Drawing for the job (mm, zero at the part's lowest x, y, z). A direction names the side the tool comes from. Give positions to 0.01 mm unless a question says otherwise; leave off trailing zeros. Order: outer loops, then holes, each group sorted by start corner. A loop starts at its lowest first (then second) coordinate and runs counter-clockwise, first axis right, second up. Notation, with made-up numbers: M 20.25,9.25 L 79.25,9.25 A29 cw 79.25,41.25 Z; hole C -23.5,14 d6. An arc over 180 degrees is marked long. One line per item, written item: value.
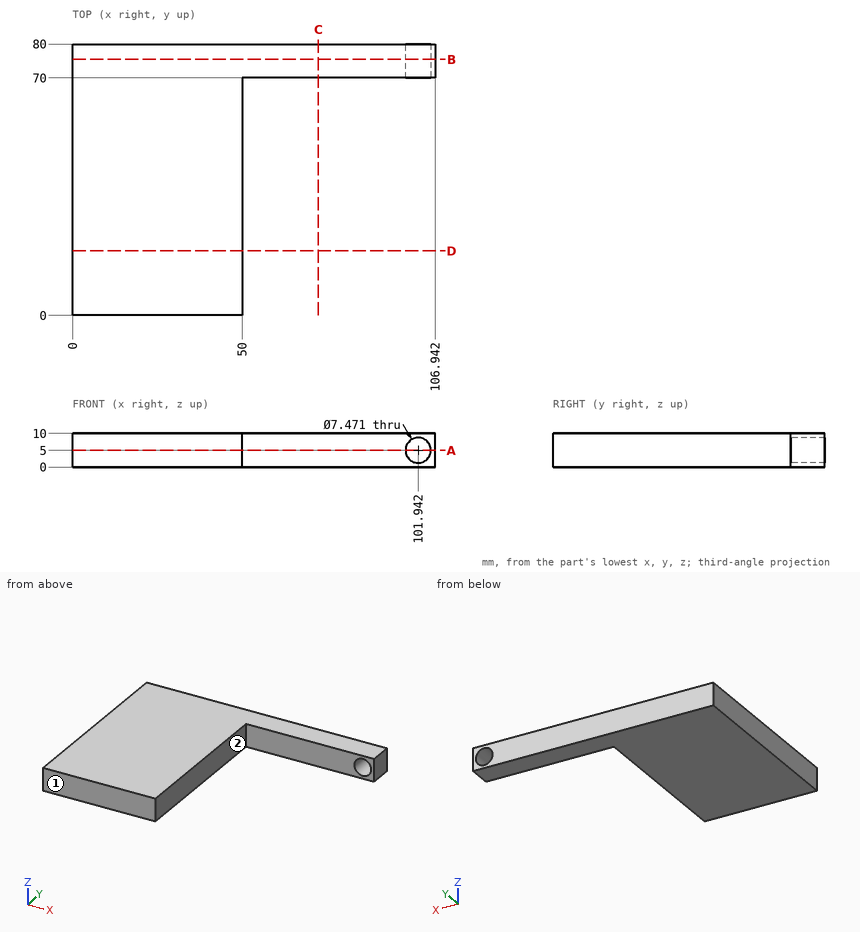
1) Saw through at B-B, the plane y = 75.5. Write the cut outline in (x, z) (1 decimal).
Check values:
outline: M 0,0 L 106.9,0 L 106.9,10 L 0,10 Z; hole C 101.9,5 d7.5
2) Saw through at D-D, the plane y = 19. Write the cut outline in (x, z), then the cut area to 3 significant figures.
Check values:
outline: M 0,0 L 50,0 L 50,10 L 0,10 Z
area: 500 mm^2
3) Saw through at C-C, the plane x = 72.5. Write the cut outline in (y, z), then the cut area to 3 significant figures.
Check values:
outline: M 70,0 L 80,0 L 80,10 L 70,10 Z
area: 100 mm^2
4) Pin check, flat tips, straight feed: pin 1 (1.5 mm diameter, centred on x = 38.5, y = 53.5, fed in from -Z); pin 2 (5 mm diameter, centred on x = 90.5, z = 5.5, fed in from -Y); pin 3 (4 mm diameter, centred on y = 13, z = 4.5, fed in from +X). Stop position of each tip, or through.
Check values:
pin 1: z = 0
pin 2: y = 70
pin 3: x = 50
5) Saw through at A-A, the plane z = 5. Write the cut outline in (x, y).
Check values:
outline: M 0,0 L 50,0 L 50,70 L 98.21,70 L 98.21,80 L 0,80 Z; M 105.68,70 L 106.94,70 L 106.94,80 L 105.68,80 Z
6) Tool access for the marked faces 1 and 2: list every direction of +Z, -Z, +X, -X, +Y, -Y with a clear straight run to the whole face (end or side of a thin tool).
Check values:
face 1: +Z, -Z, +X, -X, -Y
face 2: +Z, -Z, +X, -Y
7) Drill centre lines: probe 1 along X at (y, z) = (76.5, 5); probe 2 along X at (y, z) = (66.5, 4); probe 3 along Y at (x, z) = (97.5, 3). Where is each one in solid material? Low to high. Write a range as from..to.
Check values:
probe 1: 0..98.21, 105.68..106.94
probe 2: 0..50
probe 3: 70..80
